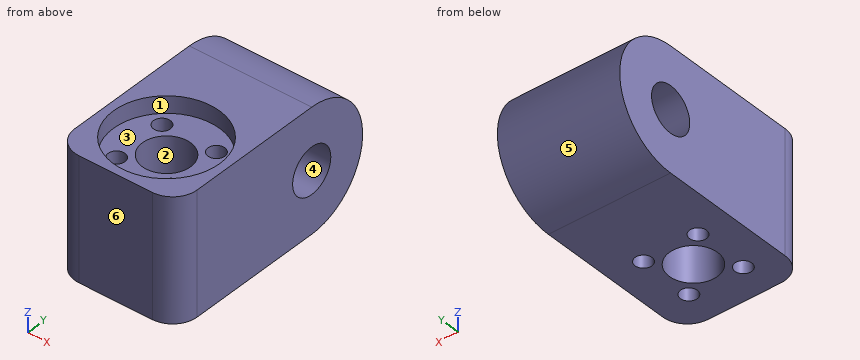
```python
from build123d import *

# Parameters (mm, degrees)
F0_W          = 25.4
F0_H          = 25.4
F1_DEPTH      = 25.4
F2_R          = 4.7625
F3_DEPTH      = 12.7
F3_DEPTH_BACK = 12.7
F4_R          = 5.08
F5_R          = 5
F5_R_2        = 1.75
F6_DEPTH      = 25.401
F7_R          = 11
F8_DEPTH      = 3.5


with BuildPart() as f1:
    # F0 (on Top) → F1 (new body)
    with BuildSketch(Plane.XY):
        Rectangle(F0_W, F0_H)
    extrude(amount=F1_DEPTH)

    # F2 (on Right) → F3 (join, two sides)
    with BuildSketch(Plane.YZ) as f3_sk:
        with BuildLine():
            Line((12.7, 0), (20.955, 0))
            ThreePointArc((20.955, 0), (33.655, 12.7), (20.955, 25.4))
            Line((20.955, 25.4), (12.7, 25.4))
            Line((12.7, 25.4), (12.7, 0))
        make_face()
        with Locations((20.955, 12.7)):
            Circle(F2_R, mode=Mode.SUBTRACT)
    extrude(amount=F3_DEPTH)
    extrude(f3_sk.sketch, amount=-F3_DEPTH_BACK)

    # F4
    f4_edges = [f1.edges().sort_by_distance(p)[0] for p in [
        (12.7, -12.7, 12.7),
        (-12.7, -12.7, 12.7),
    ]]
    fillet(f4_edges, radius=F4_R)

    # F5 (on face) → F6 (cut, through all)
    with BuildSketch(Plane.XY.offset(25.4)):
        Circle(F5_R)
        with Locations((-5.6568542495, 5.6568542495)):
            Circle(F5_R_2)
        with Locations((5.6568542495, 5.6568542495)):
            Circle(F5_R_2)
        with BuildLine():
            ThreePointArc((3.9068542495, -5.6568542495), (5.6568542495, -7.4068542495), (7.4068542495, -5.6568542495))
            ThreePointArc((7.4068542495, -5.6568542495), (5.6568542495, -3.9068542495), (3.9068542495, -5.6568542495))
        make_face()
        with Locations((-5.6568542495, -5.6568542495)):
            Circle(F5_R_2)
    extrude(amount=-F6_DEPTH, mode=Mode.SUBTRACT)

    # F7 (on face) → F8 (cut)
    with BuildSketch(Plane.XY.offset(25.4)):
        Circle(F7_R)
    extrude(amount=-F8_DEPTH, mode=Mode.SUBTRACT)


solid = f1.part
```
Build history of the part. All positions in model axes, mm. Face numbers are marked on the shaded views. A direction names the side the tool comes from. Round coordinates to 2 decimals unless told otherwise and drop trailing zeros. Write each loop counter-clockwise with the first axis right and the second up, starting at its lowest first coordinate (ties: lowest second). Pieces come first, ordered by that corner, then holes.
1) Mould opens along Z. For the marked faces 3, 4, 5 and 6 say: +Z half, -Z half, draft (parallel to the pull), parting line (faces both ways), or undercut.
2) Pin check, flat tips, straight feed: pin 1 (10 mm diameter, centred on x = -6, z = 5, fed in from +Y); pin 2 (8.5 mm diameter, centred on y = 20.955, z = 12.7, fed in from +X); pin 3 (5.5 mm diameter, centred on x = 5.66, y = 5.66, fed in from +Z); pin 4 (1 mm diameter, centred on x = 10, y = 27.5, fed in from -Z). Stop position of each tip, or through.
3) Drill centre lines: probe 1 along Y at (x, z) = (-1, 12.75); probe 2 along Y at (x, z) = (-7.25, 2.25); probe 3 along Z at (x, y) = (-7, -7). Where is each one in solid material? Low to high.
4) 3-axis set-ups, long thin cutter, end or side, ignore diameter. For the marked faces 1 and 2: which of +Z, -Z, +X, -X, +Y, -Y reach the whole face in a straight line?
5) Band-saw the part on D-D, the plane z = 1.5. List the corners of the cut face in (x, y), and give its area (3 significant figures).
6) Band-saw the part on A-A, the plane y = 0. List the corners of the cut face in (x, z), and give its area (3 significant figures).
7) Band-saw the part on B-B, the plane x = -2.5. List the corners of the cut face in (y, z) (1 decimal).
8) Band-saw the part on C-C, the plane z = 15.5. List the corners of the cut face in (x, y), and give its area (3 significant figures).
Ans:
1. face 3: +Z half
1. face 4: undercut
1. face 5: parting line
1. face 6: draft
2. pin 1: stops at y = 33.36
2. pin 2: passes through
2. pin 3: stops at z = 21.9
2. pin 4: stops at z = 1.53
3. probe 1: y = -12.7 to -4.9, 4.9 to 16.19, 25.72 to 33.65
3. probe 2: y = -12.7 to -6.38, -4.93 to 4.93, 6.38 to 28.17
3. probe 3: z = 0 to 21.9
4. face 1: +Z
4. face 2: +Z, -Z
5. outline: (-12.7, -7.62) arc R5.08 ccw to (-7.62, -12.7) - (7.62, -12.7) arc R5.08 ccw to (12.7, -7.62) - (12.7, 26.94) - (-12.7, 26.94) - close; hole circle Ø3.5 at (-5.66, -5.66); hole circle Ø3.5 at (-5.66, 5.66); hole circle Ø10 at (0, 0); hole circle Ø3.5 at (5.66, -5.66); hole circle Ø3.5 at (5.66, 5.66)
5. area: 879 mm2
6. outline: (-12.7, 0) - (-5, 0) - (-5, 21.9) - (-11, 21.9) - (-11, 25.4) - (-12.7, 25.4) - close; (5, 0) - (12.7, 0) - (12.7, 25.4) - (11, 25.4) - (11, 21.9) - (5, 21.9) - close
6. area: 349 mm2
7. outline: (-12.7, 0) - (-4.3, 0) - (-4.3, 21.9) - (-10.7, 21.9) - (-10.7, 25.4) - (-12.7, 25.4) - close; (4.3, 0) - (21, 0) arc R12.7 ccw to (21, 25.4) - (10.7, 25.4) - (10.7, 21.9) - (4.3, 21.9) - close; hole circle Ø9.5 at (21, 12.7)
8. outline: (-12.7, -7.62) arc R5.08 ccw to (-7.62, -12.7) - (7.62, -12.7) arc R5.08 ccw to (12.7, -7.62) - (12.7, 17.1) - (-12.7, 17.1) - close; (-12.7, 24.81) - (12.7, 24.81) - (12.7, 33.34) - (-12.7, 33.34) - close; hole circle Ø3.5 at (-5.66, -5.66); hole circle Ø3.5 at (-5.66, 5.66); hole circle Ø10 at (0, 0); hole circle Ø3.5 at (5.66, -5.66); hole circle Ø3.5 at (5.66, 5.66)
8. area: 846 mm2
